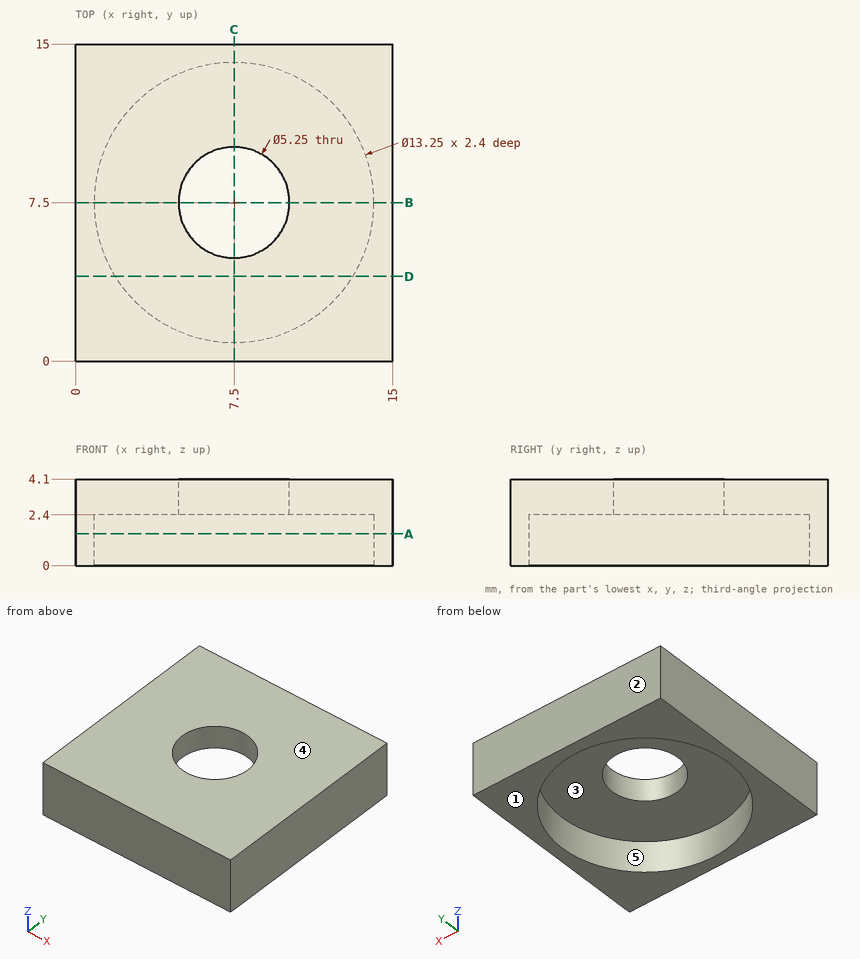
Geometry: see drawing. Coordinates: mm, zero at the bounding-box minimum. A direction names the side the tool comes from. Coordinates: 2 decimals unless noted, no trailing zeros. Order: outer loops, then holes, each group sorted by start corner. A loop starts at its lowest first (then second) coordinate and runs counter-clockwise, first axis right, second up. Notation, with made-up numbers: M 72,75 L 96,75 A29 ccw 96,97 Z; hole C -22.75,61 d6. An arc over 180 degrees is marked long. Answer in a Markdown table with one row per item. Add a question column.
Q1. Section query D-D on y = 4. Return the cut outline in (x, z) (3 decimals).
Q2. Mould query, pull axis Y, two halves, no side actions, for the marked faces 1, 2 and 3. Classes: released by +Y, released by -Y, zero draft, split by the parting line, or undercut.
Q3. Contact query for flat-ended pins moving along their axis: P1, Ø4, axis at x = 7, y = 8, coming from the -Z side; P2, Ø4, axis at x = 7.5, y = 7.5, coming from the +Z side. Output: stop coordinate, or through.
Q4. Section query A-A on z = 1.5. Return the cut outline in (x, y) (3 decimals).
Q5. Reachability of the marked faces 4 and 5 from +Z, -Z, +X, -X, +Y, -Y: full face, straight path, thin tool, end or side. Return the list, or none.
Q6. Line query: L1, parallel to Y at x = 7.5, z = 1.75 (3 decimals); L2, parallel to Y at x = 7.5, z = 3.25 (3 decimals); L3, parallel to Z at x = 3.75, y = 6. Output: solid intervals per line, ascending.
Q7. Section query B-B on y = 7.5. Return the cut outline in (x, z) (3 decimals), and give its area (3 significant figures).
Completed:
| question | item | result |
|---|---|---|
| 1 | outline | M 0,0 L 1.875,0 L 1.875,2.4 L 13.125,2.4 L 13.125,0 L 15,0 L 15,4.1 L 0,4.1 Z |
| 2 | face 1 | zero draft |
| 2 | face 2 | released by +Y |
| 2 | face 3 | undercut |
| 3 | P1 | stops at z = 2.4 |
| 3 | P2 | passes through |
| 4 | outline | M 0,0 L 15,0 L 15,15 L 0,15 Z; hole C 7.5,7.5 d13.25 |
| 5 | face 4 | +Z, +X, -X, +Y, -Y |
| 5 | face 5 | -Z |
| 6 | L1 | y = 0 to 0.875, 14.125 to 15 |
| 6 | L2 | y = 0 to 4.875, 10.125 to 15 |
| 6 | L3 | z = 2.4 to 4.1 |
| 7 | outline | M 0,0 L 0.875,0 L 0.875,2.4 L 4.875,2.4 L 4.875,4.1 L 0,4.1 Z; M 10.125,2.4 L 14.125,2.4 L 14.125,0 L 15,0 L 15,4.1 L 10.125,4.1 Z |
| 7 | area | 20.8 mm2 |
